The model under review builds one solid part; all positions refer to its coordinate system, in mm. A direction names the side the tool comes from. Coordinates: 2 decimals unless noted, no trailing zeros. Loops run counter-clockwise (first coordinate to the right, second up) from the corner with the lowest first, then second, coordinate; pieces in that order, holes last. Notation, with made-up numbers: (63, -18) - (76, -18) arc R21 ccw to (76, -9) - close; hole circle Ø8 at (-15.75, 17). An arc over 180 degrees is marked (long way). Answer in a Markdown table with one row per item. Add a question column.
(1) Machinability: for faces 4 (the flat face through (0, 2, -1)), 5 (the flat face through (-28, 12, -1)), 6 (the cylindrical face through (27.01, 10.03, -10.29)), which of the approach directions +Z, -Z, +X, -X, +Y, -Y give a long, thin tool a straight path to every point of the face, cutting with its end or side? Answer none if there is none.
(2) We need section A-A on x = 6. Write out the cut boundary in (y, z), plus the area to 3 significant figures.
(3) For P1, Ø1, axis at y = 18, z = -12, coming from the -X side; P2, Ø2, axis at x = 50, z = -25, coming from the +Y side; P3, Ø6, axis at x = 7, y = 8, coming from the -Z side; P4, Ø4, axis at x = -30.5, z = 7, coming from the +Y side, all flat-tipped, find the tip position at first contact; note any pin that passes through.
(4) We need section C-C on x = -41. Write out the cut boundary in (y, z).
(5) We need section D-D on z = -48. Write out the cut boundary in (x, y).
(6) For line 1 along Z through (x, y) = (50, 1); line 2 along Z through (x, y) = (70, 0.65); line 3 along X through (y, z) = (1.2, 57.7), list the stretches that pass through material, from the lowest coordinate up.
(7) Mouldability with a two-part tool opening along Z and no side actions: class faces 1 (the flat face through (0, 12, 43)), 2 (the flat face through (0, 12, 41)), 3 (the flat face through (28, 12, -1)) as +Z half, -Z half, draft (parallel to the pull), parting line (faces both ways), or undercut.
(8) We need section B-B on z = -35. Write out the cut boundary in (x, y), plus the area to 3 significant figures.
from build123d import *

# Parameters (mm, degrees)
ESQUISSE1_W                               = 170
ESQUISSE1_H                               = 122
BOSS_EXTRU_1_DEPTH                        = 2
TROU_POUR_TARAUDAGE_POUR_TROU_TARAUD_M3_D = 2.5
ESQUISSE4_W                               = 56
ESQUISSE4_H                               = 86
BOSS_EXTRU_2_DEPTH                        = 20
COQUE1_T                                  = -2
ENL_V_MAT_EXTRU_1_REACH                   = 132.284
ESQUISSE5_R                               = 3
ENL_V_MAT_EXTRU_2_REACH                   = 138.107
ESQUISSE6_W                               = 16
ESQUISSE6_H                               = 16
ESQUISSE6_H_2                             = 14
ENL_V_MAT_EXTRU_3_REACH                   = 132.284
ESQUISSE7_W                               = 10
ESQUISSE7_H                               = 2.54
ESQUISSE7_W_2                             = 5


with BuildPart() as part:
    # Esquisse1 → Boss.-Extru.1 (new body)
    with BuildSketch(Plane(origin=(0, 0, 0), x_dir=(1, 0, 0), z_dir=(0, 1, 0))):
        Rectangle(ESQUISSE1_W, ESQUISSE1_H)
    extrude(amount=BOSS_EXTRU_1_DEPTH)

    # Trou pour taraudage pour trou taraudé M3x0.51 (through all)
    with Locations(Plane(origin=(0, 2, 0), x_dir=(1, 0, 0), z_dir=(0, 1, 0))):
        with Locations((-50, 25), (50, 25), (50, -25), (-50, -25), (70, 57.7), (-70, -57.7), (-70, 57.7), (70, -57.7)):
            Hole(TROU_POUR_TARAUDAGE_POUR_TROU_TARAUD_M3_D / 2)

    # Esquisse4 → Boss.-Extru.2 (add)
    with BuildSketch(Plane.XZ.offset(-2)):
        Rectangle(ESQUISSE4_W, ESQUISSE4_H)
    extrude(amount=-BOSS_EXTRU_2_DEPTH)

    # Coque1
    coque1_openings = [part.faces().sort_by_distance(p)[0] for p in [
        (0, 22, 0),
    ]]
    offset(amount=COQUE1_T, openings=coque1_openings, kind=Kind.INTERSECTION)

    # Esquisse5 → Enlèv. mat.-Extru.1 (cut, up to next)
    with BuildSketch(Plane(origin=(28, 0, 0), x_dir=(0, 0, -1), z_dir=(1, 0, 0)), mode=Mode.PRIVATE) as enl_v_mat_extru_1_sk1:
        with Locations((12.5, 8)):
            Circle(ESQUISSE5_R)
    enl_v_mat_extru_1_tool1 = extrude(enl_v_mat_extru_1_sk1.sketch, amount=-ENL_V_MAT_EXTRU_1_REACH, mode=Mode.PRIVATE) & part.part
    # Esquisse5 → Enlèv. mat.-Extru.1 (cut, up to next)
    with BuildSketch(Plane(origin=(28, 0, 0), x_dir=(0, 0, -1), z_dir=(1, 0, 0)), mode=Mode.PRIVATE) as enl_v_mat_extru_1_sk2:
        with BuildLine():
            Line((-33.4, 7), (-27.4, 7))
            ThreePointArc((-27.4, 7), (-27.046446609, 6.853553391), (-26.9, 6.5))
            Line((-26.9, 6.5), (-26.9, 5.957106781))
            ThreePointArc((-26.9, 5.957106781), (-26.938060234, 5.765765065), (-27.046446609, 5.603553391))
            Line((-27.046446609, 5.603553391), (-27.503553391, 5.146446609))
            ThreePointArc((-27.503553391, 5.146446609), (-27.665765065, 5.038060234), (-27.857106781, 5))
            Line((-27.857106781, 5), (-32.942893219, 5))
            ThreePointArc((-32.942893219, 5), (-33.134234935, 5.038060234), (-33.296446609, 5.146446609))
            Line((-33.296446609, 5.146446609), (-33.753553391, 5.603553391))
            ThreePointArc((-33.753553391, 5.603553391), (-33.861939766, 5.765765065), (-33.9, 5.957106781))
            Line((-33.9, 5.957106781), (-33.9, 6.5))
            ThreePointArc((-33.9, 6.5), (-33.753553391, 6.853553391), (-33.4, 7))
        make_face()
    enl_v_mat_extru_1_tool2 = extrude(enl_v_mat_extru_1_sk2.sketch, amount=-ENL_V_MAT_EXTRU_1_REACH, mode=Mode.PRIVATE) & part.part
    # Esquisse5 → Enlèv. mat.-Extru.1 (cut, up to next)
    with BuildSketch(Plane(origin=(28, 0, 0), x_dir=(0, 0, -1), z_dir=(1, 0, 0)), mode=Mode.PRIVATE) as enl_v_mat_extru_1_sk3:
        with BuildLine():
            Line((-15.6, 9.5), (-2.4, 9.5))
            ThreePointArc((-2.4, 9.5), (-2.046446609, 9.353553391), (-1.9, 9))
            Line((-1.9, 9), (-1.9, 7))
            ThreePointArc((-1.9, 7), (-2.046446609, 6.646446609), (-2.4, 6.5))
            Line((-2.4, 6.5), (-2.696630825, 6.5))
            ThreePointArc((-2.696630825, 6.5), (-2.922638662, 6.446004998), (-3.099833323, 6.295681832))
            Line((-3.099833323, 6.295681832), (-3.900166677, 5.204318168))
            ThreePointArc((-3.900166677, 5.204318168), (-4.077361338, 5.053995002), (-4.303369175, 5))
            Line((-4.303369175, 5), (-13.696630825, 5))
            ThreePointArc((-13.696630825, 5), (-13.922638662, 5.053995002), (-14.099833323, 5.204318168))
            Line((-14.099833323, 5.204318168), (-14.900166677, 6.295681832))
            ThreePointArc((-14.900166677, 6.295681832), (-15.077361338, 6.446004998), (-15.303369175, 6.5))
            Line((-15.303369175, 6.5), (-15.6, 6.5))
            ThreePointArc((-15.6, 6.5), (-15.953553391, 6.646446609), (-16.1, 7))
            Line((-16.1, 7), (-16.1, 9))
            ThreePointArc((-16.1, 9), (-15.953553391, 9.353553391), (-15.6, 9.5))
        make_face()
    enl_v_mat_extru_1_tool3 = extrude(enl_v_mat_extru_1_sk3.sketch, amount=-ENL_V_MAT_EXTRU_1_REACH, mode=Mode.PRIVATE) & part.part
    add(enl_v_mat_extru_1_tool1.solids().sort_by_distance((28, 8, -12.5))[0], mode=Mode.SUBTRACT)
    add(enl_v_mat_extru_1_tool2.solids().sort_by_distance((28, 6.025513, 30.4))[0], mode=Mode.SUBTRACT)
    add(enl_v_mat_extru_1_tool3.solids().sort_by_distance((28, 7.376996, 9))[0], mode=Mode.SUBTRACT)

    # Esquisse6 → Enlèv. mat.-Extru.2 (cut, up to next)
    with BuildSketch(Plane(origin=(0, 0, -43), x_dir=(-1, 0, 0), z_dir=(0, 0, -1)), mode=Mode.PRIVATE) as enl_v_mat_extru_2_sk1:
        with Locations((17.5, 11.6)):
            Rectangle(ESQUISSE6_W, ESQUISSE6_H)
    enl_v_mat_extru_2_tool1 = extrude(enl_v_mat_extru_2_sk1.sketch, amount=-ENL_V_MAT_EXTRU_2_REACH, mode=Mode.PRIVATE) & part.part
    # Esquisse6 → Enlèv. mat.-Extru.2 (cut, up to next)
    with BuildSketch(Plane(origin=(0, 0, -43), x_dir=(-1, 0, 0), z_dir=(0, 0, -1)), mode=Mode.PRIVATE) as enl_v_mat_extru_2_sk2:
        with Locations((0, 11.6)):
            Rectangle(ESQUISSE6_W, ESQUISSE6_H)
    enl_v_mat_extru_2_tool2 = extrude(enl_v_mat_extru_2_sk2.sketch, amount=-ENL_V_MAT_EXTRU_2_REACH, mode=Mode.PRIVATE) & part.part
    # Esquisse6 → Enlèv. mat.-Extru.2 (cut, up to next)
    with BuildSketch(Plane(origin=(0, 0, -43), x_dir=(-1, 0, 0), z_dir=(0, 0, -1)), mode=Mode.PRIVATE) as enl_v_mat_extru_2_sk3:
        with Locations((-18, 10.6)):
            Rectangle(ESQUISSE6_W, ESQUISSE6_H_2)
    enl_v_mat_extru_2_tool3 = extrude(enl_v_mat_extru_2_sk3.sketch, amount=-ENL_V_MAT_EXTRU_2_REACH, mode=Mode.PRIVATE) & part.part
    add(enl_v_mat_extru_2_tool1.solids().sort_by_distance((-17.5, 11.6, -43))[0], mode=Mode.SUBTRACT)
    add(enl_v_mat_extru_2_tool2.solids().sort_by_distance((0, 11.6, -43))[0], mode=Mode.SUBTRACT)
    add(enl_v_mat_extru_2_tool3.solids().sort_by_distance((18, 10.6, -43))[0], mode=Mode.SUBTRACT)

    # Esquisse7 → Enlèv. mat.-Extru.3 (cut, up to next)
    with BuildSketch(Plane.ZY.offset(28), mode=Mode.PRIVATE) as enl_v_mat_extru_3_sk1:
        with Locations((12.251607125, 13.425584158)):
            Rectangle(ESQUISSE7_W, ESQUISSE7_H)
    enl_v_mat_extru_3_tool1 = extrude(enl_v_mat_extru_3_sk1.sketch, amount=-ENL_V_MAT_EXTRU_3_REACH, mode=Mode.PRIVATE) & part.part
    # Esquisse7 → Enlèv. mat.-Extru.3 (cut, up to next)
    with BuildSketch(Plane.ZY.offset(28), mode=Mode.PRIVATE) as enl_v_mat_extru_3_sk2:
        with Locations((24.751607125, 13.425584158)):
            Rectangle(ESQUISSE7_W_2, ESQUISSE7_H)
    enl_v_mat_extru_3_tool2 = extrude(enl_v_mat_extru_3_sk2.sketch, amount=-ENL_V_MAT_EXTRU_3_REACH, mode=Mode.PRIVATE) & part.part
    add(enl_v_mat_extru_3_tool1.solids().sort_by_distance((-28, 13.425584, 12.251607))[0], mode=Mode.SUBTRACT)
    add(enl_v_mat_extru_3_tool2.solids().sort_by_distance((-28, 13.425584, 24.751607))[0], mode=Mode.SUBTRACT)


solid = part.part
Outcome:
| question | item | result |
|---|---|---|
| 1 | face 4 | +Y |
| 1 | face 5 | +Z, -Z, -X, +Y |
| 1 | face 6 | +X |
| 2 | outline | (0, -61) - (2, -61) - (2, -43) - (3.6, -43) - (3.6, -41) - (2, -41) - (2, 41) - (22, 41) - (22, 43) - (2, 43) - (2, 61) - (0, 61) - close; (19.6, -43) - (22, -43) - (22, -41) - (19.6, -41) - close |
| 2 | area | 292 mm² |
| 3 | P1 | x = -28 |
| 3 | P2 | through |
| 3 | P3 | z = -43 |
| 3 | P4 | y = 2 |
| 4 | outline | (0, -61) - (2, -61) - (2, 61) - (0, 61) - close |
| 5 | outline | (-85, 0) - (85, 0) - (85, 2) - (-85, 2) - close |
| 6 | line 1 | -61 to -26.25, -23.75 to 23.75, 26.25 to 61 |
| 6 | line 2 | -61 to -58.95, -56.45 to 56.45, 58.95 to 61 |
| 6 | line 3 | -85 to -71.25, -68.75 to 68.75, 71.25 to 85 |
| 7 | face 1 | +Z half |
| 7 | face 2 | undercut |
| 7 | face 3 | draft |
| 8 | outline | (-85, 0) - (85, 0) - (85, 2) - (28, 2) - (28, 22) - (26, 22) - (26, 2) - (-26, 2) - (-26, 22) - (-28, 22) - (-28, 2) - (-85, 2) - close |
| 8 | area | 420 mm² |
